Build history of the part. All positions in model axes, mm. Face numbers are marked on the shaded views. A direction names the side the tool comes from. Give positions to 0.01 mm unless a question says otherwise; leave off trailing zeros. Order: outer loops, then holes, each group sorted by start corner. A loop starts at its lowest first (then second) coordinate and runs counter-clockwise, first axis right, second up. Notation, with made-up numbers: M 75,26 L 84,26 A24 ccw 84,58 Z; hole C 10,-33.75 d4. An arc over 180 degrees is marked long. One line per item, written item: value. Start each with the question number.
from build123d import *

# Parameters (mm, degrees)
SKETCH1_R                         = 23
LENGTH_DEPTH                      = 565
SKETCH2_R                         = 23
HIP_JOINT_DEPTH                   = 100
TIBIA_AXIS_REACH                  = 576.242
TIBIA_AXIS_END_RADIUS             = 23
SKETCH3_R                         = 9.071418029
TIBIA_AXIS_DIRECTION_2_REACH      = 576.242
TIBIA_AXIS_DIRECTION_2_END_RADIUS = 23


with BuildPart() as part:
    # Sketch1 → Length (new body)
    with BuildSketch(Plane(origin=(0, 0, 0), x_dir=(0, 0, -1), z_dir=(1, 0, 0))):
        Circle(SKETCH1_R)
    extrude(amount=LENGTH_DEPTH)

    # Sketch2 → Hip joint (add)
    with BuildSketch(Plane.XY):
        with Locations(Location((0, 0, 0), (0, 0, 270))):
            Circle(SKETCH2_R)
    extrude(amount=HIP_JOINT_DEPTH)

    # Tibia axis: up to this cylinder (the profile starts inside it)
    tibia_axis_end = Plane(origin=(567.07131, 0, 0), z_dir=(-1, 0, 0)) * Cylinder(TIBIA_AXIS_END_RADIUS, 1199.484, mode=Mode.PRIVATE)
    # Sketch3 → Tibia axis (cut, up to the surface)
    with BuildSketch(Plane.XY, mode=Mode.PRIVATE) as tibia_axis_sk1:
        with Locations((567.071310444, 0)):
            Circle(SKETCH3_R)
    tibia_axis_tool1 = extrude(tibia_axis_sk1.sketch, amount=-TIBIA_AXIS_REACH, mode=Mode.PRIVATE) & tibia_axis_end
    add(tibia_axis_tool1.solids().sort_by_distance((567.07131, 0, 0))[0], mode=Mode.SUBTRACT)

    # Tibia axis direction 2: up to this cylinder (the profile starts inside it)
    tibia_axis_direction_2_end = Plane(origin=(567.07131, 0, 0), z_dir=(-1, 0, 0)) * Cylinder(TIBIA_AXIS_DIRECTION_2_END_RADIUS, 1199.484, mode=Mode.PRIVATE)
    # Sketch3 → Tibia axis direction 2 (cut, up to the surface)
    with BuildSketch(Plane.XY, mode=Mode.PRIVATE) as tibia_axis_direction_2_sk1:
        with Locations((567.071310444, 0)):
            Circle(SKETCH3_R)
    tibia_axis_direction_2_tool1 = extrude(tibia_axis_direction_2_sk1.sketch, amount=TIBIA_AXIS_DIRECTION_2_REACH, mode=Mode.PRIVATE) & tibia_axis_direction_2_end
    add(tibia_axis_direction_2_tool1.solids().sort_by_distance((567.07131, 0, 0))[0], mode=Mode.SUBTRACT)


solid = part.part
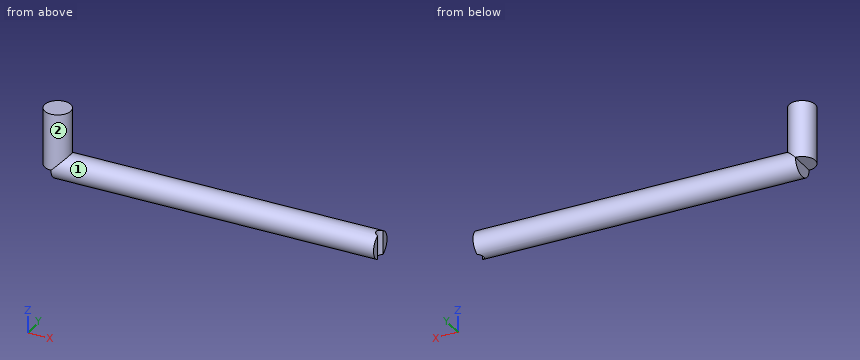
1) Drop flat-ended pins along their axis: P1, Ø8, axis at x = 203.5, y = 16, coming from the +Z side; P2, Ø12, axis at y = -18.5, z = 41.5, coming from the -X side; P3, Ø5, axis at x = 461, y = 12, coming from the +Z side. Give the stop position or say it passes through.
2) Tool access for the marked faces 1 and 2: list every direction of +Z, -Z, +X, -X, +Y, -Y with a clear straight run to the whole face (end or side of a thin tool).
3) Drill centre lines: line 1 (Z direction, x = 53.5, y = -1.5); line 2 (Z direction, x = 438, y = 1). Where is each one in solid material? Low to high.
4) Slice it at A-A (y = 0). List the corners of the cut face in (x, z).
5) Slice it at B-B (x = 494). List the corners of the cut face in (y, z).
6) Slice it at D-D (z = -5). List the corners of the cut face in (x, y), plus the area to 3 significant figures.
Results list:
1. P1: stops at z = 19.62
1. P2: stops at x = -19.31
1. P3: stops at z = 20.95
2. face 1: +X
2. face 2: +Z
3. line 1: z = -22.95 to 22.95
3. line 2: z = -22.98 to 22.98
4. outline: M -23,0 L 0,0 L 0,-23 L 558,-23 L 558,23 L 23,23 L 23,100 L -23,100 Z
5. outline: C 0,0 d46
6. outline: M 0,-22.45 L 565,-22.45 L 565,-8.83 A9.07 cw 565,8.83 L 565,22.45 L 0,22.45 Z
6. area: 25,300 mm²
